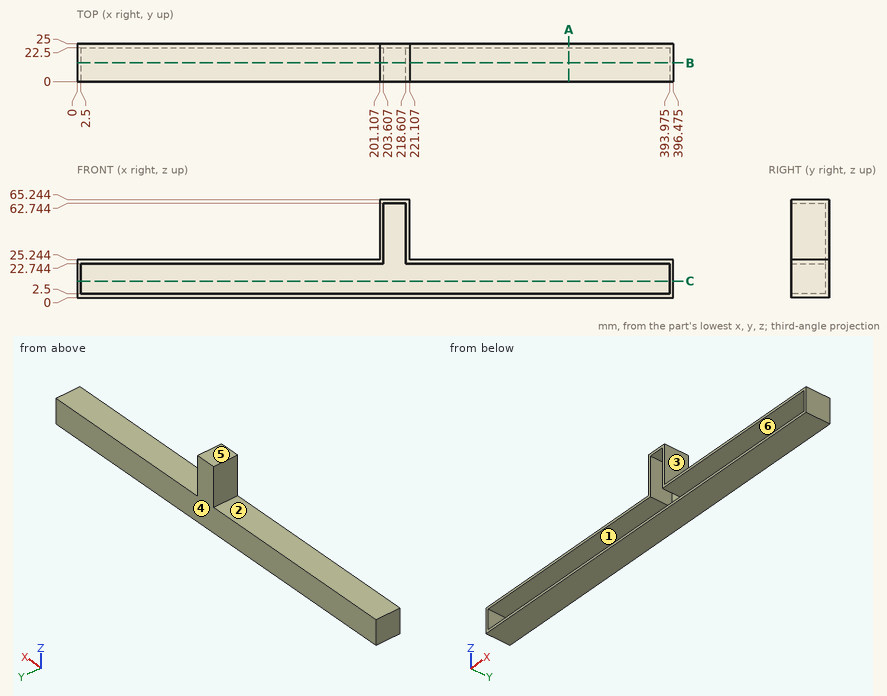
For this review, use the dimensioned drawing (mm, ordinates from the lowest corner) and the shaded views. A direction names the side the tool comes from. Coordinates: 2 decimals unless noted, no trailing zeros. Loops run counter-clockwise (first coordinate to the right, second up) from the corner with the lowest first, then second, coordinate; pieces in that order, holes last. Notation, with made-up numbers: (-21, 60) -> (32, 60) arc R20 ccw to (32, 97) -> close; hole circle Ø8 at (11.5, -39.75). An arc over 180 degrees is marked (long way). Use a Markdown table: item, result. Add a question column.
Item 1: Clearance check with flat-ended pins moving along their axes: P1, Ø2, axis at y = 14.5, z = 34.5, coming from the -X side; P2, Ø1, axis at x = 302, y = 21, coming from the +Z side; P3, Ø6, axis at x = 157, z = 12, coming from the -Y side. State where each tip first meets the part, or that it passes through.
Item 2: Machinability: for the marked faces 1, 2 and 3, which of the approach directions +Z, -Z, +X, -X, +Y, -Y give a long, thin tool a straight path to every point of the face, cutting with its end or side? Answer none if there is none.
Item 3: We need section A-A, the plane x = 327. Write out the cut boundary in (y, z) (1 decimal).
Item 4: Wall thickness on L1, parallel to X at y = 11, z = 16 (1 decimal); L2, parallel to Z at x = 73, y = 3.5 (1 decimal); L3, parallel to X at y = 3.75, z = 32.5: over which ranges is each line inside the solid? List them lowest first. Write a range as from..to.
Item 5: We need section B-B, the plane y = 12.5. Write out the cut boundary in (x, z) (1 decimal).
Item 6: The part is to be moulded in two halves that separate along Z. For the marked faces 4, 5 and 6, say which applies: +Z half, -Z half, draft (parallel to the pull), parting line (faces both ways), or undercut.
Item 7: We need section C-C, the plane z = 11. Write out the cut boundary in (x, y) (1 decimal).
Numbers:
| question | item | result |
|---|---|---|
| 1 | P1 | stops at x = 201.11 |
| 1 | P2 | stops at z = 25.24 |
| 1 | P3 | stops at y = 22.5 |
| 2 | face 1 | -Y |
| 2 | face 2 | +Z, -X, +Y, -Y |
| 2 | face 3 | +Z, +X, +Y, -Y |
| 3 | outline | (0, 0) -> (25, 0) -> (25, 25.2) -> (0, 25.2) -> (0, 22.7) -> (22.5, 22.7) -> (22.5, 2.5) -> (0, 2.5) -> close |
| 4 | L1 | x = 0..2.5, 394..396.5 |
| 4 | L2 | z = 0..2.5, 22.7..25.2 |
| 4 | L3 | x = 201.11..203.61, 218.61..221.11 |
| 5 | outline | (0, 0) -> (396.5, 0) -> (396.5, 25.2) -> (221.1, 25.2) -> (221.1, 65.2) -> (201.1, 65.2) -> (201.1, 25.2) -> (0, 25.2) -> close; hole (2.5, 2.5) -> (394, 2.5) -> (394, 22.7) -> (218.6, 22.7) -> (218.6, 62.7) -> (203.6, 62.7) -> (203.6, 22.7) -> (2.5, 22.7) -> close |
| 6 | face 4 | draft |
| 6 | face 5 | +Z half |
| 6 | face 6 | undercut |
| 7 | outline | (0, 0) -> (2.5, 0) -> (2.5, 22.5) -> (394, 22.5) -> (394, 0) -> (396.5, 0) -> (396.5, 25) -> (0, 25) -> close |
